```python
from build123d import *

# Parameters (mm, degrees)
SKETCH1_R                                       = 15
BOSS_EXTRUDE1_DEPTH                             = 10
CSK_FOR_M6_FLAT_HEAD_MACHINE_SCREW2_D           = 6
CSK_FOR_M6_FLAT_HEAD_MACHINE_SCREW2_CSINK_D     = 12.6
CSK_FOR_M6_FLAT_HEAD_MACHINE_SCREW2_CSINK_ANGLE = 90
SKETCH6_W                                       = 51
SKETCH6_H                                       = 25.5
CUT_EXTRUDE1_DEPTH                              = 10


with BuildPart() as part:
    # Sketch1 → Boss-Extrude1 (new body)
    with BuildSketch(Plane(origin=(0, 0, 0), x_dir=(1, 0, 0), z_dir=(0, 1, 0))):
        with BuildLine():
            Line((-155, 175), (155, 175))
            ThreePointArc((155, 175), (169.142135624, 169.142135624), (175, 155))
            Line((175, 155), (175, -155))
            ThreePointArc((175, -155), (169.142135624, -169.142135624), (155, -175))
            Line((155, -175), (-155, -175))
            ThreePointArc((-155, -175), (-169.142135624, -169.142135624), (-175, -155))
            Line((-175, -155), (-175, 155))
            ThreePointArc((-175, 155), (-169.142135624, 169.142135624), (-155, 175))
        make_face()
        with Locations(Location((-109.601551084, 109.601551084, 0), (0, 0, 270))):
            Circle(SKETCH1_R, mode=Mode.SUBTRACT)
        with Locations(Location((109.601551084, 109.601551084, 0), (0, 0, 270))):
            Circle(SKETCH1_R, mode=Mode.SUBTRACT)
        with Locations(Location((-109.601551084, -109.601551084, 0), (0, 0, 270))):
            Circle(SKETCH1_R, mode=Mode.SUBTRACT)
        with Locations(Location((109.601551084, -109.601551084, 0), (0, 0, 270))):
            Circle(SKETCH1_R, mode=Mode.SUBTRACT)
    extrude(amount=BOSS_EXTRUDE1_DEPTH)

    # CSK for M6 Flat Head Machine Screw2 (through all)
    with Locations(Plane(origin=(160, 0, -160), x_dir=(0, 0, -1), z_dir=(0, -1, 0))):
        with Locations((0, 0), (-160, 0), (-320, 0), (-320, -160), (-320, -320), (-160, -320), (0, -320), (0, -160)):
            CounterSinkHole(CSK_FOR_M6_FLAT_HEAD_MACHINE_SCREW2_D / 2, CSK_FOR_M6_FLAT_HEAD_MACHINE_SCREW2_CSINK_D / 2, counter_sink_angle=CSK_FOR_M6_FLAT_HEAD_MACHINE_SCREW2_CSINK_ANGLE)

    # Sketch6 → Cut-Extrude1 (cut)
    with BuildSketch(Plane(origin=(0, 10, 0), x_dir=(1, 0, 0), z_dir=(0, 1, 0))):
        with Locations((98.666512481, -12.75)):
            Rectangle(SKETCH6_W, SKETCH6_H)
    extrude(amount=-CUT_EXTRUDE1_DEPTH, mode=Mode.SUBTRACT)


solid = part.part
```
Can you work these out from the model? Positions are in its coordinate system, mm. A direction names the side the tool comes from. Coordinates: 2 decimals unless noted, no trailing zeros. Return JSON: item names as keys, results as strings.
Q1. I'm going to push a flat-ended pin straight in: pin 1 Ø8 at (x, z) = (-160, 0) entering from -Y. Where does the tip first touch, or does it pass through?
Computed values:
{"pin 1": "stops at y = 2.3"}
Q2. On a 3-axis mill with a long thin cutter (end or side, diameter ignored), from which of +Z, -Z, +X, -X, +Y, -Y can I reach the whole of each face in a straight line? I mean faces 5 (the flat face through (98, 5, 0)), 6 (the conical face through (-163.085, 3.14, 159.315)). Say none if no direction works.
Computed values:
{"face 5": "+Y, -Y", "face 6": "-Y"}
Q3. If we section it at A-A (y = 6.5): Count the separate pieces of the cut face and the enclosed holes in it, then the cut area to 3 significant figures.
Computed values:
{"separate pieces": "1", "enclosed holes": "13", "area": "118,000 mm2"}
Q4. Thinking about a two-plate mould opening in Z: for faces 1 (the flat face through (2, 10, -2)), 2 (the cylindrical face through (-169.297, 4.93, -168.986)), 3 (the flat face through (2, 5, 175)), 4 (the flat face through (73.167, 5, 13)), which applies, +Z half, -Z half, draft (parallel to the pull), parting line (faces both ways), or undercut?
Computed values:
{"face 1": "draft", "face 2": "-Z half", "face 3": "+Z half", "face 4": "undercut"}
Q5. Please list where these lines run through material, in increasing order: L1, parallel to Z at x = 0, y = 8.75; L2, parallel to Z at x = -121, y = 2; L3, parallel to Z at x = -160, y = 7.25. Write a range as from..to.
Computed values:
{"L1": "z = -175..-163, -157..157, 163..175", "L2": "z = -175..-119.35, -99.85..99.85, 119.35..175", "L3": "z = -174.36..-163, -157..-3, 3..157, 163..174.36"}
